Build history of the part. All positions in model axes, mm. A direction names the side the tool comes from. Give positions to 0.01 mm unless a question says otherwise; leave off trailing zeros. Order: outer loops, then holes, each group sorted by start corner. A loop starts at its lowest first (then second) coordinate and runs counter-clockwise, first axis right, second up. Notation, with made-up numbers: M -3,70.5 L 48,70.5 A15 ccw 48,94.5 Z; hole C -29,-15 d6. An arc over 180 degrees is marked long. Answer as CSV lines item,"result".
from build123d import *

# Parameters (mm, degrees)
F0_R     = 22.606
F1_DEPTH = 17.145


# Not quite as in the source:
# - a feature names something its author has since deleted; it is built from what else it names


with BuildPart() as f1:
    # F0 (on Front) → F1 (new body)
    with BuildSketch(Plane.XZ):
        with BuildLine():
            ThreePointArc((1.778, 34.8797124558), (25.3165190636, 24.0588754413), (34.925, 0))
            ThreePointArc((34.925, 0), (-24.0588754413, -25.3165190636), (-1.778, 34.8797124558))
            Line((-1.778, 34.8797124558), (-1.778, 47.591799094))
            ThreePointArc((-1.778, 47.591799094), (-7.4944029118, 47.0316335034), (-13.1017966196, 45.7873732631))
            ThreePointArc((-13.1017966196, 45.7873732631), (-47.1633558849, -6.6150197786), (0, -47.625))
            Line((0, -47.625), (88.9, -35.306))
            ThreePointArc((88.9, -35.306), (124.206, 0), (88.9, 35.306))
            Line((88.9, 35.306), (12.3385861516, 45.9152244904))
            Line((12.3385861516, 45.9152244904), (1.778, 47.37862))
            Line((1.778, 47.37862), (1.778, 34.8797124558))
        make_face()
        with Locations((88.9, 0)):
            Circle(F0_R, mode=Mode.SUBTRACT)
        with BuildLine():
            ThreePointArc((-13.1017966196, 45.7873732631), (-7.4944029118, 47.0316335034), (-1.778, 47.591799094))
            Line((-1.778, 47.591799094), (-1.778, 60.96))
            Line((-1.778, 60.96), (-13.1017966196, 60.96))
            Line((-13.1017966196, 60.96), (-13.1017966196, 45.7873732631))
        make_face()
        Polygon((1.778, 60.96), (1.778, 47.37862), (12.3385861516, 45.9152244904), (12.3385861516, 60.96), align=None)
    extrude(amount=F1_DEPTH)


solid = f1.part
Item 1: 3-axis set-ups, long thin cutter, end or side, ignore diameter. For faces 4 (the flat face through (1.778, -8, 48)), 5 (the flat face through (12.339, -8, 53)), 6 (the flat face through (43.83, -8.45, -41.55)), 7 (the flat face through (-13.102, -8, 53)), 8 (the flat face through (-7, -8, 60.96)): which of +Z, -Z, +X, -X, +Y, -Y reach the whole face in a straight line?
Geometry says:
face 4,"+Z, +Y, -Y"
face 5,"+Z, +X, +Y, -Y"
face 6,"-Z, +X, +Y, -Y"
face 7,"+Z, -X, +Y, -Y"
face 8,"+Z, +X, -X, +Y, -Y"
Item 2: Drop flat-ended pins along their axis: pin 1 (4 mm diameter, centred on x = 21, y = -15.5, fed in from +Z); pin 2 (6 mm diameter, centred on x = 51, y = -12, fed in from -Z); pin 3 (6 mm diameter, centred on x = 72, y = -13, fed in from +Z); pin 4 (4 mm diameter, centred on x = -20.5, z = -24, fed in from +Y). Give the stop position or say it passes through.
Geometry says:
pin 1,"stops at z = 44.99"
pin 2,"stops at z = -40.97"
pin 3,"stops at z = 38.06"
pin 4,"passes through"
Item 3: Band-saw the part on D-D (z = -12). Give the cut face in (x, y) (3 decimals), and give its area (3 significant figures).
Geometry says:
outline,"M -46.088,-17.145 L -32.799,-17.145 L -32.799,0 L -46.088,0 Z; M 32.799,-17.145 L 69.742,-17.145 L 69.742,0 L 32.799,0 Z; M 108.058,-17.145 L 122.104,-17.145 L 122.104,0 L 108.058,0 Z"
area,"1,100 mm2"
Item 4: Probe line 1 along X through (y, z) = (-3.5, 53); line 2 along X through (y, z) = (-5, 0.5); line 3 along X through (y, z) = (-10.75, -11). List the from-to ranges inside material, lowest first. Write a range as from..to.
Geometry says:
line 1,"x = -13.1..-1.78, 1.78..12.34"
line 2,"x = -47.62..-34.92, 34.92..66.3, 111.5..124.2"
line 3,"x = -46.34..-33.15, 33.15..69.15, 108.65..122.45"
Item 5: Band-saw the part on A-A (y = -13). Give the cut face in (x, z) (3 decimals).
Geometry says:
outline,"M -13.102,45.787 A47.625 ccw 0,-47.625 L 88.9,-35.306 A35.306 ccw 88.9,35.306 L 12.339,45.915 L 12.339,60.96 L 1.778,60.96 L 1.778,34.88 A34.925 cw long -1.778,34.88 L -1.778,60.96 L -13.102,60.96 Z; hole C 88.9,0 d45.212"
Item 6: Band-saw the part on B-B (z = 48.5). Give the cut face in (x, y) (3 decimals), and give its area (3 significant figures).
Geometry says:
outline,"M -13.102,-17.145 L -1.778,-17.145 L -1.778,0 L -13.102,0 Z; M 1.778,-17.145 L 12.339,-17.145 L 12.339,0 L 1.778,0 Z"
area,"375 mm2"
Item 7: Band-saw the part on C-C (x = 95.5). Give the cut face in (y, z) (3 decimals), and give its area (3 significant figures).
Geometry says:
outline,"M -17.145,-34.684 L 0,-34.684 L 0,-21.621 L -17.145,-21.621 Z; M -17.145,21.621 L 0,21.621 L 0,34.684 L -17.145,34.684 Z"
area,"448 mm2"
Item 8: Pull direction X, two halves, no side cores. Call faces 1 (the flat face through (7, -8, 60.96)), 2 (the flat face through (-1.778, -8, 48)), 3 (the flat face through (51.155, -8.452, 40.536)): released by +X, released by -X, zero draft, split by the parting line, or undercut.
Geometry says:
face 1,"zero draft"
face 2,"undercut"
face 3,"released by +X"
